```python
from build123d import *

# Parameters (mm, degrees)
BOSS_EXTRU_1_DEPTH           = 8
ESQUISSE2_R                  = 7.15
ENL_V_MAT_EXTRU_1_DEPTH      = 265.732643435
R_VOLUTION1_ANGLE            = 180
ESQUISSE4_R                  = 30.35
ENL_V_MAT_EXTRU_2_DEPTH      = 4
ENL_V_MAT_EXTRU_3_DEPTH      = 268.017031292
ENL_V_MAT_EXTRU_3_DEPTH_BACK = 268.017031292
ESQUISSE5_R                  = 7.15


with BuildPart() as part:
    # Esquisse1 → Boss.-Extru.1 (new, symmetric)
    with BuildSketch(Plane(origin=(0, 0, 0), x_dir=(1, 0, 0), z_dir=(0, 1, 0))):
        with BuildLine():
            Line((-232.15, 30.35), (232.15, 30.35))
            ThreePointArc((232.15, 30.35), (262.5, 0), (232.15, -30.35))
            Line((232.15, -30.35), (-232.15, -30.35))
            ThreePointArc((-232.15, -30.35), (-262.5, 0), (-232.15, 30.35))
        make_face()
    extrude(amount=BOSS_EXTRU_1_DEPTH, both=True)

    # Esquisse2 → Enlèv. mat.-Extru.1 (cut, through all)
    with BuildSketch(Plane(origin=(0, 8, 0), x_dir=(1, 0, 0), z_dir=(0, 1, 0))):
        with Locations(Location((232.15, 0, 0), (0, 0, 270))):
            Circle(ESQUISSE2_R)
    extrude(amount=-ENL_V_MAT_EXTRU_1_DEPTH, mode=Mode.SUBTRACT)

    # Esquisse3 → Révolution1 (revolve)
    with BuildSketch(Plane(origin=(0, 8, 0), x_dir=(1, 0, 0), z_dir=(0, 1, 0))):
        with BuildLine():
            Line((-232.15, 30.35), (-232.15, -30.35))
            ThreePointArc((-232.15, -30.35), (-262.5, 0), (-232.15, 30.35))
        make_face()
    r_volution1 = revolve(axis=Axis((-232.15, 8, -30.35), (0, 0, -1)), revolution_arc=R_VOLUTION1_ANGLE)

    # Symétrie1: Révolution1 across plane
    add(r_volution1.mirror(Plane.ZX))

    # Esquisse4 → Enlèv. mat.-Extru.2 (cut, symmetric)
    with BuildSketch(Plane(origin=(0, 0, 0), x_dir=(1, 0, 0), z_dir=(0, 1, 0))):
        with Locations((-232.15, 0)):
            Circle(ESQUISSE4_R)
    extrude(amount=ENL_V_MAT_EXTRU_2_DEPTH, both=True, mode=Mode.SUBTRACT)

    # Esquisse5 → Enlèv. mat.-Extru.3 (cut, two sides: drawn at the far end of the back side and taken through both)
    with BuildSketch(Plane(origin=(0, 0, 0), x_dir=(1, 0, 0), z_dir=(0, 1, 0)).offset(-ENL_V_MAT_EXTRU_3_DEPTH_BACK)):
        with Locations(Location((-232.15, 0, 0), (0, 0, 270))):
            Circle(ESQUISSE5_R)
    extrude(amount=ENL_V_MAT_EXTRU_3_DEPTH + ENL_V_MAT_EXTRU_3_DEPTH_BACK, mode=Mode.SUBTRACT)


solid = part.part
```
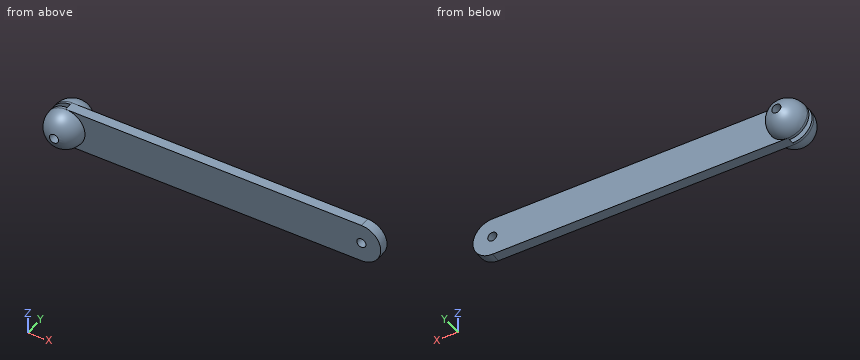
Could you check a few things on this model? Use its own coordinates, in mm. Round coordinates to 2 decimals unless told otherwise and drop trailing zeros. Loops run counter-clockwise (first coordinate to the right, second up) from the corner with the lowest first, then second, coordinate; pieces in that order, holes last.
Q1. I want a section at D-D (y = 19). Write out the boundary of the cut face in (x, z).
Q2. I want a section at B-B (x = -142). Write out the boundary of the cut face in (y, z).
Q3. Please list where these lines run through material, in increasing order: L1, parallel to X at y = 2.75, z = 0; L2, parallel to Z at x = 232, y = 4; L3, parallel to Y at x = 23.5, z = 8.5.
Q4. I want a section at A-A (z = 0). Write out the boundary of the cut face in (x, y), and give its area (3 significant figures).
Q5. I want a section at C-C (z = -26). Write out the boundary of the cut face in (x, y), and give its area (3 significant figures).
Q6. For P1, Ø8, axis at y = 12, z = -13, coming from the -X side; P2, Ø1, axis at x = 28, z = 10, coming from the -Y side; P3, Ø1, axis at y = -2.5, z = -4.5, coming from the +X side; P4, Ø8.5, axis at x = -232.15, z = 0, coming from the +Y side, each with a flat end and sliding along its axis, tell me the tip position at first contact or that it passes through.
Answer below:
1. outline: circle Ø56.57 at (-232.15, 0); hole circle Ø14.3 at (-232.15, 0)
2. outline: (-8, -30.35) - (8, -30.35) - (8, 30.35) - (-8, 30.35) - close
3. L1: x = -201.8 to 225, 239.3 to 262.5
3. L2: z = -30.35 to -7.15, 7.15 to 30.35
3. L3: y = -8 to 8
4. outline: (-262.5, -8) arc R30.35 ccw to (-239.3, -37.5) - (-239.3, -4) - (-262.5, -4) - close; (-262.5, 4) - (-239.3, 4) - (-239.3, 37.5) arc R30.35 ccw to (-262.5, 8) - close; (-225, -37.5) arc R30.35 ccw to (-201.8, -8) - (225, -8) - (225, 8) - (-201.8, 8) arc R30.35 ccw to (-225, 37.5) - (-225, 4) - (-201.8, 4) - (-201.8, -4) - (-225, -4) - close; (239.3, -8) - (262.5, -8) - (262.5, 8) - (239.3, 8) - close
4. area: 9,610 mm2
5. outline: (-247.81, -8) arc R15.66 ccw to (-216.49, -8) - (247.81, -8) - (247.81, 8) - (-216.49, 8) arc R15.66 ccw to (-247.81, 8) - (-247.81, 4) - (-216.49, 4) - (-216.49, -4) - (-247.81, -4) - close
5. area: 8,450 mm2
6. P1: stops at x = -260.94
6. P2: stops at y = -8
6. P3: stops at x = 262.24
6. P4: passes through
